Design review of the part built by this model. Coordinates are the model's own, in mm. Face numbers are marked on the shaded views. A direction names the side the tool comes from. Round coordinates to 2 decimals unless told otherwise and drop trailing zeros. Order: outer loops, then holes, each group sorted by start corner. A loop starts at its lowest first (then second) coordinate and runs counter-clockwise, first axis right, second up. Notation, with made-up numbers: (-35.5, 42) - (-27.5, 42) arc R20 cw to (-27.5, 81) - close; hole circle Ø8 at (-24.75, 13). An arc over 180 degrees is marked (long way). Answer as a JSON object with one key per item and string values. Group by question number.
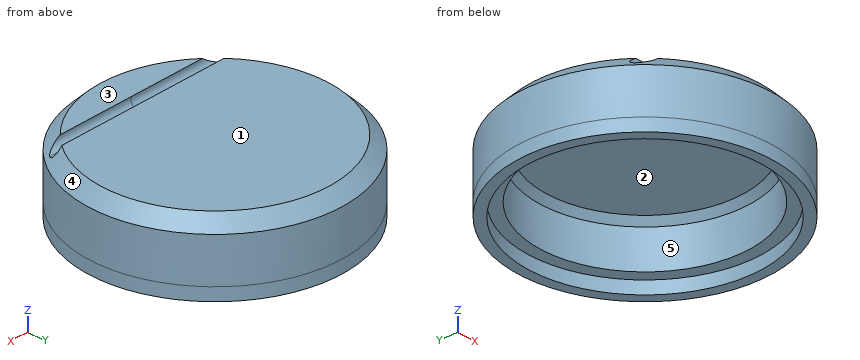
from build123d import *

# Parameters (mm, degrees)
SKETCH1_R               = 10
SKETCH1_R_2             = 8.25
BOSS_EXTRUDE1_DEPTH     = 4.5
SKETCH1_3_R             = 8.25
BOSS_EXTRUDE2_DEPTH     = 1
SKETCH2_R               = 10
SKETCH2_R_2             = 9.2
BOSS_EXTRUDE3_DEPTH     = 1
CHAMFER1_SIZE           = 1
CHAMFER2_SIZE           = 0.5
SKETCH4_R               = 0.5
CUT_EXTRUDE3_DEPTH      = 11
CUT_EXTRUDE3_DEPTH_BACK = 11


with BuildPart() as part:
    # Sketch1 → Boss-Extrude1 (new body)
    with BuildSketch(Plane.XY):
        Circle(SKETCH1_R)
        Circle(SKETCH1_R_2, mode=Mode.SUBTRACT)
    extrude(amount=-BOSS_EXTRUDE1_DEPTH)

    # Sketch1<3> → Boss-Extrude2 (add)
    with BuildSketch(Plane.XY):
        Circle(SKETCH1_3_R)
    extrude(amount=-BOSS_EXTRUDE2_DEPTH)

    # Sketch2 → Boss-Extrude3 (add)
    with BuildSketch(Plane(origin=(0, 0, -4.5), x_dir=(-1, 0, 0), z_dir=(0, 0, -1))):
        Circle(SKETCH2_R)
        Circle(SKETCH2_R_2, mode=Mode.SUBTRACT)
    extrude(amount=BOSS_EXTRUDE3_DEPTH)

    # Chamfer1
    chamfer1_edges = [part.edges().sort_by_distance(p)[0] for p in [
        (-10, 0, 0),
    ]]
    chamfer(chamfer1_edges, length=CHAMFER1_SIZE)

    # Chamfer2
    chamfer2_edges = [part.edges().sort_by_distance(p)[0] for p in [
        (-8.25, 0, -1),
    ]]
    chamfer(chamfer2_edges, length=CHAMFER2_SIZE)

    # Sketch4 → Cut-Extrude3 (cut, two sides)
    with BuildSketch(Plane(origin=(0, 0, 0), x_dir=(0, 0, -1), z_dir=(1, 0, 0))) as cut_extrude3_sk:
        with Locations((0.2, -6.15)):
            Circle(SKETCH4_R)
    extrude(amount=CUT_EXTRUDE3_DEPTH, mode=Mode.SUBTRACT)
    extrude(cut_extrude3_sk.sketch, amount=-CUT_EXTRUDE3_DEPTH_BACK, mode=Mode.SUBTRACT)


solid = part.part
1. To check wall thickness, follow line 1 (Y direction, x = 0, z = -3.2); line 2 (Y direction, x = 0, z = -4.8); line 3 (Z direction, x = 7.5, y = -1.5). State the ranges of each line that lie inside material, in increasing order. Write a range as from..to.
2. Mouldability with a two-part tool opening along Y and no side actions: class the marked faces 3, 4 and 5 as pulls with the +Y half, pulls with the -Y half, needs draft (parallel to the pull), parting line crosses it, or undercut.
3. Clearance check with flat-ended pins moving along their axes: P1, Ø5.5, axis at x = 4, y = 2, coming from the -Z side; P2, Ø3, axis at x = 7, z = -4.5, coming from the -Y side; P3, Ø1, axis at x = -5.5, z = -5, coming from the -Y side. State where each tip first meets the part, or that it passes through.
4. Tool access review of the marked faces 1 and 2: name each direction out of +Z, -Z, +X, -X, +Y, -Y from which nothing blocks a thin tool from reaching the whole face with its end or side.
5. Take a section at A-A, the plane y = 0. Give the boundary of the cut face in (x, z), then the cut area to 3 significant figures.
6. Take a section at B-B, the plane z = -2.1. Give the boundary of the cut face in (x, y).
Response values:
{
 "1": {"line 1": "-10..-8.25, 8.25..10", "line 2": "-10..-9.2, 9.2..10", "line 3": "-1..0"},
 "2": {"face 3": "needs draft", "face 4": "parting line crosses it", "face 5": "undercut"},
 "3": {"P1": "z = -1", "P2": "y = -8.35", "P3": "y = -8.66"},
 "4": {"face 1": "+Z, +X, -X, +Y, -Y", "face 2": "-Z"},
 "5": {"outline": "(-10, -5.5) - (-9.2, -5.5) - (-9.2, -4.5) - (-8.25, -4.5) - (-8.25, -1.5) - (-7.75, -1) - (7.75, -1) - (8.25, -1.5) - (8.25, -4.5) - (9.2, -4.5) - (9.2, -5.5) - (10, -5.5) - (10, -1) - (9, 0) - (-9, 0) - (-10, -1) - close", "area": "33.1 mm2"},
 "6": {"outline": "circle Ø20 at (0, 0); hole circle Ø16.5 at (0, 0)"}
}
